Here's how the part is built. I have some questions about the finished solid (model axes, mm). Face numbers are marked on the shaded views. A direction names the side the tool comes from. Round coordinates to 2 decimals unless told otherwise and drop trailing zeros. Order: outer loops, then holes, each group sorted by start corner. A loop starts at its lowest first (then second) coordinate and runs counter-clockwise, first axis right, second up. Notation, with made-up numbers: M -25,45 L -18,45 A29 cw -18,72 Z; hole C 19.25,70 d6. An arc over 180 degrees is marked long. Answer as CSV lines item,"result". Start each with the question number.
```python
from build123d import *

# Parameters (mm, degrees)
F1_DEPTH = 11.1125


# Not quite as in the source:
# - a length typed as a fraction of an inch, garbled in the dataset ("3 / 203.2 mm" for 3/8 in), is restored


with BuildPart() as f1:
    # F0 (on Top) → F1 (new body)
    with BuildSketch(Plane.XY):
        with BuildLine():
            ThreePointArc((-0.1411418198, 20.1985444874), (-5.0054503986, 18.2564119782), (-9.2097157612, 15.1327075437))
            ThreePointArc((-9.2097157612, 15.1327075437), (-10.6205392688, 11.8246856933), (-10.2093555033, 8.2519613206))
            Line((-10.2093555033, 8.2519613206), (-12.369341217, 7.1464567445))
            Line((-12.369341217, 7.1464567445), (-12.369341217, 4.6386048198))
            Line((-12.369341217, 4.6386048198), (-12.369341217, 4.5682978211))
            ThreePointArc((-12.369341217, 4.5682978211), (-15.5930977879, 3.1185654947), (-17.7027139134, 0.2823972963))
            ThreePointArc((-17.7027139134, 0.2823972963), (-21.0452825194, -1.0603738309), (-23.1384971151, -3.9919692741))
            ThreePointArc((-23.1384971151, -3.9919692741), (-23.9954710425, -8.6613028545), (-23.5336683691, -13.3861117065))
            ThreePointArc((-23.5336683691, -13.3861117065), (-19.6562098094, -16.4130421994), (-15.0192606046, -18.054899429))
            ThreePointArc((-15.0192606046, -18.054899429), (-11.4338171794, -17.7079201351), (-8.5996589687, -15.484556372))
            ThreePointArc((-8.5996589687, -15.484556372), (-5.0294162563, -15.0523544446), (-2.1409380715, -12.9098966718))
            Line((-2.1409380715, -12.9098966718), (0, -14.2561570176))
            Line((0, -14.2561570176), (1.9696742658, -12.9098966718))
            ThreePointArc((1.9696742658, -12.9098966718), (4.9392756736, -15.0084468105), (8.560301624, -15.3410370587))
            ThreePointArc((8.560301624, -15.3410370587), (13.367982191, -13.3015402533), (17.4874793738, -10.0916987285))
            ThreePointArc((17.4874793738, -10.0916987285), (18.16772005, -4.8427956267), (17.6633565687, 0.4259166096))
            ThreePointArc((17.6633565687, 0.4259166096), (15.4847616458, 3.3168082822), (12.1560195839, 4.739132713))
            Line((12.1560195839, 4.739132713), (12.1560195839, 7.1464567445))
            Line((12.1560195839, 7.1464567445), (9.9960338703, 8.2519613206))
            ThreePointArc((9.9960338703, 8.2519613206), (10.4072176357, 11.8246856933), (8.9963941282, 15.1327075437))
            ThreePointArc((8.9963941282, 15.1327075437), (4.7823081966, 18.3053860292), (-0.1411418198, 20.1985444874))
        make_face()
    extrude(amount=F1_DEPTH)


solid = f1.part
```
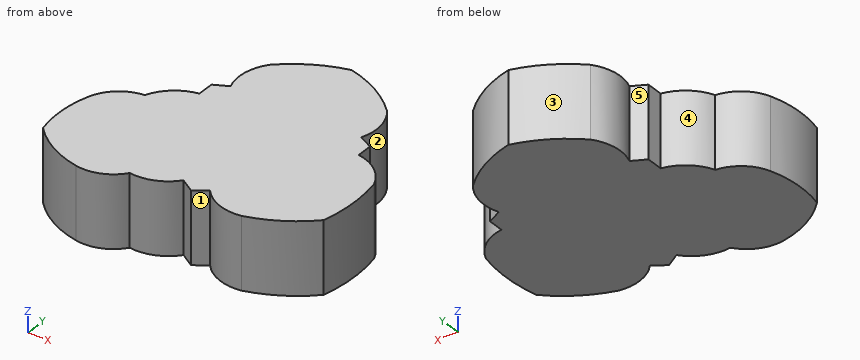
Item 1: If we section it at B-B on x = 4.5: Please give me the cut outline in (y, z), and give its area (3 significant figures).
Item 2: For P1, Ø1.5, axis at y = 14.5, z = 2, coming from the -X side; P2, Ø5, axis at x = 11, z = 1, coming from the -Y side; P3, Ø0.8, axis at y = 6, z = 3, coming from the -X side, each with a flat end and sliding along its axis, tell me the tip position at first contact or that it passes through.
Item 3: If we section it at A-A on z = 5.5: Please give me the cut outline in (x, y), and give its area (3 significant figures).
Item 4: We'd pull the mould along X, two halves only. Please class the marked faces 1, 2 and 3: pulls with the +X half, pulls with the -X half, needs draft (parallel to the pull), parting line crosses it, or undercut.
Item 5: If I drill on line 1 along Y through (x, z) = (5, 0.5); line 2 along X through (y, z) = (6.5, 4.75); line 3 along X through (y, z) = (-1, 4.75), over which ranges is the centre line in solid material (lowest first)?
Item 6: If we section it at C-C on y = 18.5: Please give me the cut outline in (x, z), and give its area (3 significant figures).
Item 7: Which directions (+Z, -Z, +X, -X, +Y, -Y) give clear straight access to the entire face, cutting with the end or side of a thin tool? Please do the marked faces 4 and 5.
Geometry says:
1,outline,"M -14.83,0 L 18.46,0 L 18.46,11.11 L -14.83,11.11 Z"
1,area,"370 mm²"
2,P1,"x = -10.05"
2,P2,"y = -15.35"
2,P3,"x = -12.37"
3,outline,"M -23.53,-13.39 A15.32 ccw -15.02,-18.05 A6.42 ccw -8.6,-15.48 A7.02 ccw -2.14,-12.91 L 0,-14.26 L 1.97,-12.91 A7.02 ccw 8.56,-15.34 A20.09 ccw 17.49,-10.09 A23.64 ccw 17.66,0.43 A7.02 ccw 12.16,4.74 L 12.16,7.15 L 10,8.25 A7.02 ccw 9,15.13 A19.02 ccw -0.14,20.2 A20.27 ccw -9.21,15.13 A7.02 ccw -10.21,8.25 L -12.37,7.15 L -12.37,4.57 A7.02 ccw -17.7,0.28 A6.42 ccw -23.14,-3.99 A17.07 ccw Z"
3,area,"1,050 mm²"
4,face 1,"undercut"
4,face 2,"pulls with the +X half"
4,face 3,"pulls with the -X half"
5,line 1,"-15.03 to 18.18"
5,line 2,"-12.37 to 12.16"
5,line 3,"-20.97 to 17.92"
6,outline,"M -4.56,0 L 4.42,0 L 4.42,11.11 L -4.56,11.11 Z"
6,area,"99.8 mm²"
7,face 4,"+Z, -Z, -X, +Y"
7,face 5,"+Z, -Z, -X"
